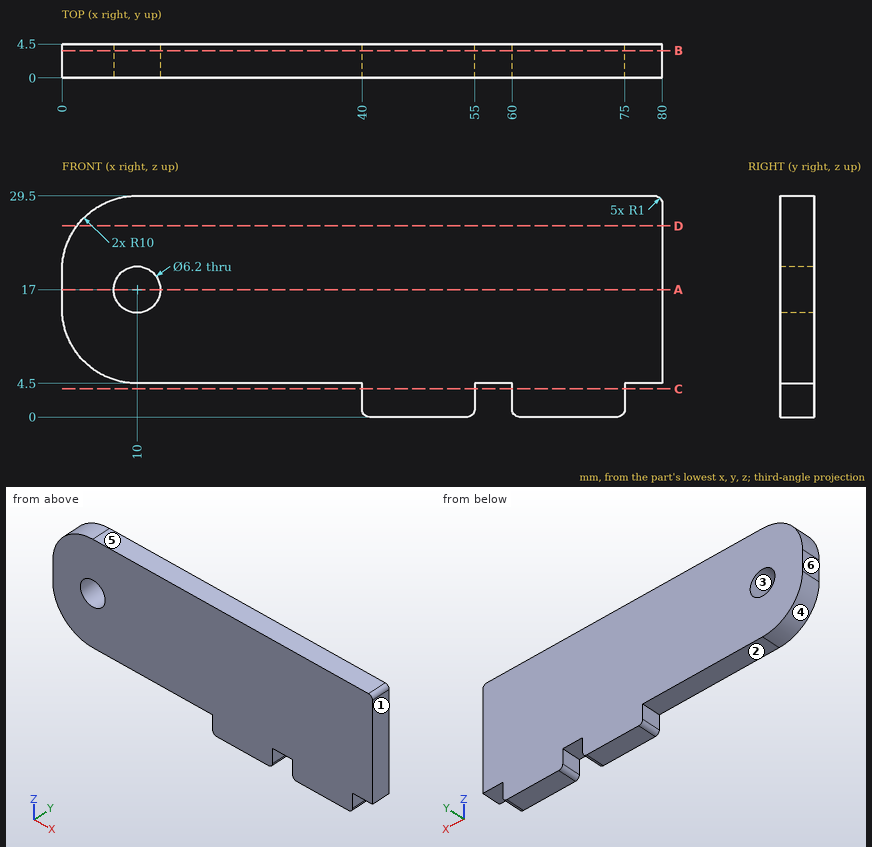
Answer from the drawing. Dimensions are ordinates in mm from the lowest x, y and z of the part. A direction names the side the tool comes from. Coordinates: 2 decimals unless noted, no trailing zeros. Write each loop counter-clockwise with the first axis right and the second up, starting at its lowest first coordinate (ties: lowest second). Pieces come first, ordered by that corner, then holes. Notation, with made-up numbers: M 13,28.25 L 29,28.25 A16 cw 29,57.25 Z; hole C 35.5,-30 d6. An arc over 180 degrees is marked long. Put each result on its own line as item: value. Start each with the question number.
1. A cutting plane is placed at C-C on z = 3.75. Write down the section's boundary in (x, y).
2. For a pull along Z with two mould halves and no side action, classify the marked faces 3, 4, 5 and 6 as pulls with the +Z half, pulls with the -Z half, needs draft (parallel to the pull), parting line crosses it, or undercut.
3. A cutting plane is placed at B-B on y = 3.6. Write down the section's boundary in (x, z), then the cut area to 3 significant figures.
4. A cutting plane is placed at A-A on z = 17. Write down the section's boundary in (x, y).
5. Consider line 1 (X direction, y = 3.35, z = 4); line 2 (X direction, y = 1.5, z = 17); line 3 (Z direction, x = 11, y = 3.95). Determine where each line is inside the solid, lowest interval first. Write a range as from..to.
6. A cutting plane is placed at D-D on z = 25.5. Write down the section's boundary in (x, y).
7. Flat-ended cylindrical pins translate along their axes: P1, Ø1, axis at y = 3, z = 2, coming from the -X side; P2, Ø1.3, axis at x = 23.5, y = 1, coming from the -Z side; P3, Ø3.5, axis at x = 10, z = 17, coming from the +Y side. Find the tip coordinate at first contact, or state that the pin passes through.
8. Which of the six approach directions +Z, -Z, +X, -X, +Y, -Y give full straight-line access (tool end or side, diameter ignored) to the marked faces 1 and 2?
Resolved:
1. outline: M 40,0 L 55,0 L 55,4.5 L 40,4.5 Z; M 60,0 L 75,0 L 75,4.5 L 60,4.5 Z
2. face 3: undercut
2. face 4: pulls with the -Z half
2. face 5: pulls with the +Z half
2. face 6: needs draft
3. outline: M 0,14.5 A10 ccw 10,4.5 L 40,4.5 L 40,1 A1 ccw 41,0 L 54,0 A1 ccw 55,1 L 55,4.5 L 60,4.5 L 60,1 A1 ccw 61,0 L 74,0 A1 ccw 75,1 L 75,4.5 L 80,4.5 L 80,28.5 A1 ccw 79,29.5 L 10,29.5 A10 ccw 0,19.5 Z; hole C 10,17 d6.2
3. area: 2,060 mm2
4. outline: M 0,0 L 6.9,0 L 6.9,4.5 L 0,4.5 Z; M 13.1,0 L 80,0 L 80,4.5 L 13.1,4.5 Z
5. line 1: x = 40..55, 60..75
5. line 2: x = 0..6.9, 13.1..80
5. line 3: z = 4.5..14.07, 19.93..29.5
6. outline: M 2,0 L 80,0 L 80,4.5 L 2,4.5 Z
7. P1: stops at x = 40
7. P2: stops at z = 4.5
7. P3: passes through
8. face 1: +Z, -Z, +X, +Y, -Y
8. face 2: -Z, -X, +Y, -Y
